The listing builds one solid part. Answer for the finished solid, in the listing's coordinates (mm). Face numbers are marked on the shaded views. A direction names the side the tool comes from. Give positions to 0.01 mm unless a question says otherwise; leave off trailing zeros. Order: outer loops, then holes, each group sorted by start corner. A loop starts at its lowest first (then second) coordinate and runs counter-clockwise, first axis right, second up. Notation, with made-up numbers: (-38.5, 1) - (-30.5, 1) arc R10 cw to (-30.5, 14) - close; hole circle Ø6 at (-23.75, -5). An arc over 180 degrees is marked (long way). Answer in a Markdown table with one row per item. Add a question column.
```python
from build123d import *

# Parameters (mm, degrees)
SKETCH1_W                = 120.65
SKETCH1_H                = 25.4
SKETCH1_R                = 2.38125
BOSS_EXTRUDE1_DEPTH      = 6.35
SKETCH2_R                = 2.38125
CUT_EXTRUDE1_DEPTH       = 6.35
BOSS_EXTRUDE2_DEPTH      = 38.1
BOSS_EXTRUDE2_DEPTH_BACK = 38.1
SKETCH3_W                = 5.08
SKETCH3_H                = 25.4
SKETCH4_R                = 2.38125
CUT_EXTRUDE2_DEPTH       = 130.203386179
FILLET1_R                = 2.54
FILLET2_R                = 7.62
FILLET3_R                = 12.7


with BuildPart() as part:
    # Sketch1 → Boss-Extrude1 (new body)
    with BuildSketch(Plane(origin=(0, 0, 0), x_dir=(1, 0, 0), z_dir=(0, 1, 0))):
        Rectangle(SKETCH1_W, SKETCH1_H)
        with Locations(Location((47.625, 0, 0), (0, 0, 270))):
            Circle(SKETCH1_R, mode=Mode.SUBTRACT)
    extrude(amount=BOSS_EXTRUDE1_DEPTH)

    # Sketch2 → Cut-Extrude1 (cut)
    with BuildSketch(Plane(origin=(0, 6.35, 0), x_dir=(1, 0, 0), z_dir=(0, 1, 0))):
        with Locations(Location((-41.275, 0, 0), (0, 0, 270))):
            Circle(SKETCH2_R)
    extrude(amount=-CUT_EXTRUDE1_DEPTH, mode=Mode.SUBTRACT)

    # Sketch3 → Boss-Extrude2 (add, two sides: drawn at the far end of the back side and taken through both)
    with BuildSketch(Plane(origin=(0, 6.35, 0), x_dir=(1, 0, 0), z_dir=(0, 1, 0)).offset(-BOSS_EXTRUDE2_DEPTH_BACK)):
        with Locations((-57.785, 0)):
            Rectangle(SKETCH3_W, SKETCH3_H)
    extrude(amount=BOSS_EXTRUDE2_DEPTH + BOSS_EXTRUDE2_DEPTH_BACK)

    # Sketch4 → Cut-Extrude2 (cut, through all)
    with BuildSketch(Plane.ZY.offset(60.325)):
        with Locations((0, 25.4)):
            Circle(SKETCH4_R)
        with Locations((0, -25.4)):
            Circle(SKETCH4_R)
        with Locations((0, 38.1)):
            Circle(SKETCH4_R)
    extrude(amount=-CUT_EXTRUDE2_DEPTH, mode=Mode.SUBTRACT)

    # Fillet1
    fillet1_edges = [part.edges().sort_by_distance(p)[0] for p in [
        (-55.245, 0, 0),
        (-55.245, 6.35, 0),
    ]]
    fillet(fillet1_edges, radius=FILLET1_R)

    # Fillet2
    fillet2_edges = [part.edges().sort_by_distance(p)[0] for p in [
        (-57.785, -31.75, -12.7),
        (-57.785, -31.75, 12.7),
        (-57.785, 44.45, 12.7),
        (-57.785, 44.45, -12.7),
    ]]
    fillet(fillet2_edges, radius=FILLET2_R)

    # Fillet3
    fillet3_edges = [part.edges().sort_by_distance(p)[0] for p in [
        (60.325, 3.175, 12.7),
        (60.325, 3.175, -12.7),
    ]]
    fillet(fillet3_edges, radius=FILLET3_R - 0.0001)  # a hair under: the kernel refuses the full size


solid = part.part
```
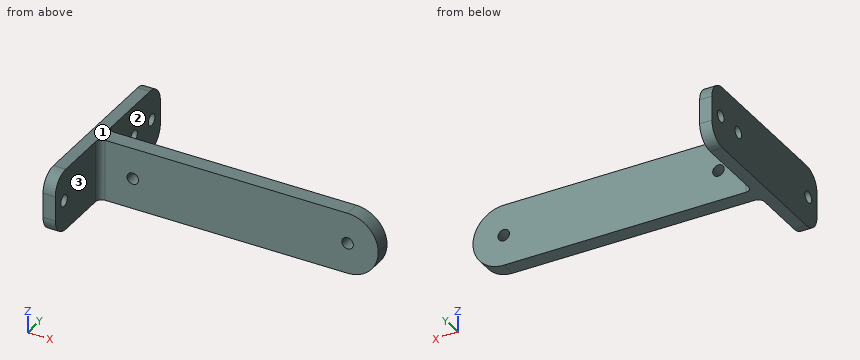
(1) Find section A-A, the plane y = 25.4. Write down the section's boundary in (x, z) (3 decimals), plus the area to 3 significant figures.
(2) Find section C-C, the plane x = -6. Write down the section's boundary in (y, z).
(3) Straight lines are drawn through the part: line 1 (X direction, y = 2.5, z = 0) (3 decimals); line 2 (Y direction, x = -57.55, z = 0); line 3 (Y direction, x = -26, z = -6.5). For each, find the intervals that lie inside material, in ascending order.
(4) Each of these flat-tipped pins is pushed along its axis until it touches: P1, Ø12.5, axis at x = -12, z = -4.5, coming from the +Y side; P2, Ø3, axis at x = 19.5, z = -0.5, coming from the +Y side; P3, Ø8, axis at y = -8, z = 0.5, coming from the +X side (3 decimals); P4, Ø6, axis at y = 38.1, z = 0, coming from the -X side (3 decimals). Where does it stop, or does it pass through?
(5) Find section D-D, the plane y = 38.1. Write down the section's boundary in (x, z) (3 decimals), plus the area to 3 significant figures.
(6) For the marked faces 1, 2 and 3, determine the directions among +Z, -Z, +X, -X, +Y, -Y from which every point of the face is accessible in a straight line to the end or side of a thin tool.
(7) Find section B-B, the plane y = -8. Write down the section's boundary in (x, z) (3 decimals).
Answer key:
| question | item | result |
|---|---|---|
| 1 | outline | (-60.325, -12.7) - (-55.245, -12.7) - (-55.245, -2.381) - (-60.325, -2.381) - close; (-60.325, 2.381) - (-55.245, 2.381) - (-55.245, 12.7) - (-60.325, 12.7) - close |
| 1 | area | 105 mm² |
| 2 | outline | (0, -12.7) - (6.35, -12.7) - (6.35, 12.7) - (0, 12.7) - close |
| 3 | line 1 | -60.325 to -43.656, -38.894 to 45.244, 50.006 to 60.325 |
| 3 | line 2 | -31.75 to -27.78, -23.02 to 23.02, 27.78 to 35.72, 40.48 to 44.45 |
| 3 | line 3 | 0 to 6.35 |
| 4 | P1 | y = 6.35 |
| 4 | P2 | y = 6.35 |
| 4 | P3 | x = -55.245 |
| 4 | P4 | x = -60.325 |
| 5 | outline | (-60.325, -12.593) - (-55.245, -12.593) - (-55.245, -2.381) - (-60.325, -2.381) - close; (-60.325, 2.381) - (-55.245, 2.381) - (-55.245, 12.593) - (-60.325, 12.593) - close |
| 5 | area | 104 mm² |
| 6 | face 1 | +Z, +X, -X, +Y, -Y |
| 6 | face 2 | +Z, -Z, +X, +Y |
| 6 | face 3 | +Z, -Z, +X, -Y |
| 7 | outline | (-60.325, -12.7) - (-55.245, -12.7) - (-55.245, 12.7) - (-60.325, 12.7) - close |
